Answer from the drawing. Dimensions are ordinates in mm from the lowest x, y and z of the part. A direction names the side the tool comes from. Give positions to 0.01 mm unless a question says otherwise; leave off trailing zeros. Write each loop counter-clockwise with the first axis right and the second up, starting at its lowest first coordinate (ties: lowest second). Pieces come first, ordered by that corner, then holes. Notation, with made-up numbers: (44.5, 55.25) -> (84.5, 55.25) arc R27 ccw to (84.5, 83.25) -> close; hole circle Ø2 at (3, 26). An arc over 180 degrees is marked (long way). Put each result on its own line as item: value. Start each with the question number.
1) Find the intervals of material crossed by line 1 along Y through (x, z) = (57, 10) (1 decimal); line 2 along Y through (x, z) = (55.95, 10.75) (1 decimal); line 3 along Z through (x, y) = (57, 18) (1 decimal), in increasing order. Write a range as from..to.
2) For the marked faces 1, 2 and 3, determine the directions among +Z, -Z, +X, -X, +Y, -Y from which every point of the face is accessible in a straight line to the end or side of a thin tool.
3) A cutting plane is placed at B-B (y = 27). Write down the section's boundary in (x, z), then the cut area to 3 significant figures.
4) A cutting plane is placed at A-A (z = 18.5). Write down the section's boundary in (x, y), then the cut area to 3 significant figures.
5) A cutting plane is placed at D-D (z = 3). Write down the section's boundary in (x, y), then the cut area to 3 significant figures.
6) A cutting plane is placed at C-C (x = 50). Write down the section's boundary in (y, z).
7) Flat-ended cylindrical pins translate along their axes: pin 1 Ø2.5 at (y, z) = (5.5, 11) entering from +X; pin 2 Ø0.6 at (x, y) = (3, 12.5) entering from -Z; pin 3 Ø4 at (y, z) = (5.08, 26.25) entering from -X. Find the tip coordinate at first contact, or state that the pin passes through.
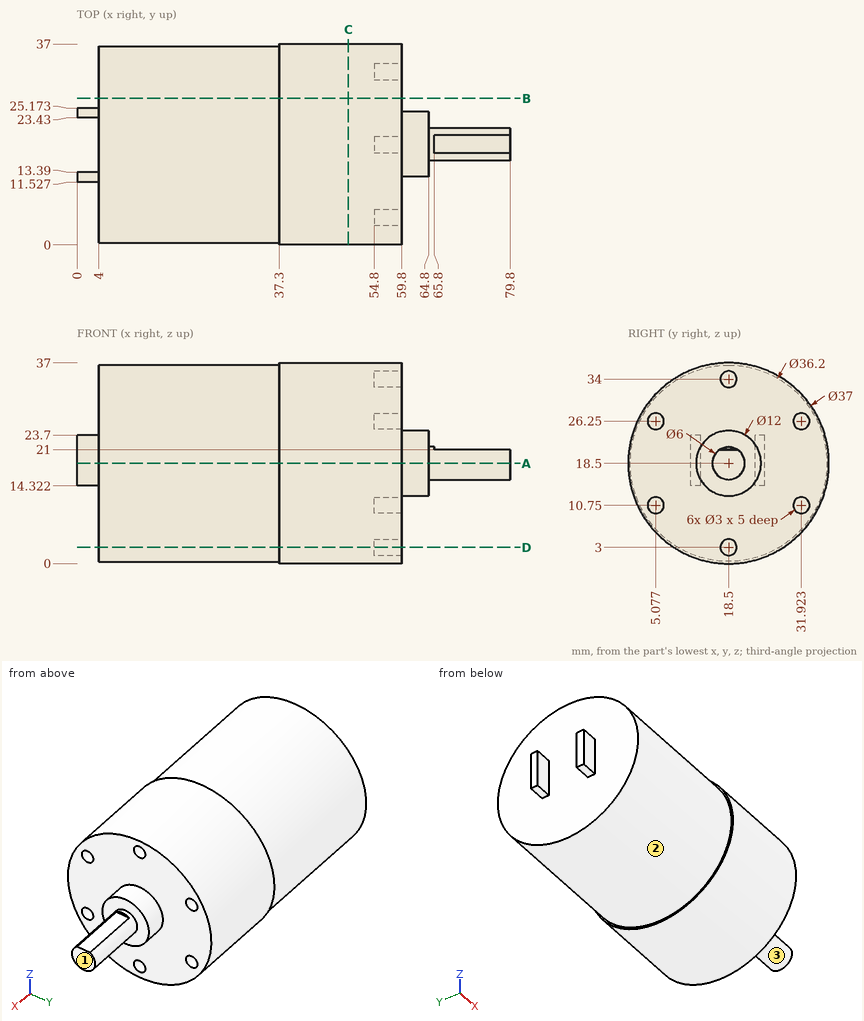
Reply:
1. line 1: y = 2.1..3.8, 6.4..30.6, 33.2..34.9
1. line 2: y = 1.7..3.6, 6.6..30.4, 33.4..35.3
1. line 3: z = 0..1.6, 4.4..32.6, 35.4..37
2. face 1: +Z, -Z, +X, +Y, -Y
2. face 2: -X
2. face 3: +X
3. outline: (4, 2.52) -> (37.3, 2.52) -> (37.3, 2.07) -> (59.8, 2.07) -> (59.8, 34.93) -> (37.3, 34.93) -> (37.3, 34.48) -> (4, 34.48) -> close
3. area: 1,800 mm2
4. outline: (0, 11.53) -> (4, 11.53) -> (4, 0.4) -> (37.3, 0.4) -> (37.3, 0) -> (59.8, 0) -> (59.8, 12.5) -> (64.8, 12.5) -> (64.8, 15.5) -> (79.8, 15.5) -> (79.8, 21.5) -> (64.8, 21.5) -> (64.8, 24.5) -> (59.8, 24.5) -> (59.8, 37) -> (37.3, 37) -> (37.3, 36.6) -> (4, 36.6) -> (4, 25.17) -> (0, 25.17) -> (0, 23.43) -> (4, 23.43) -> (4, 13.39) -> (0, 13.39) -> close
4. area: 2,200 mm2
5. outline: (4, 9.15) -> (37.3, 9.15) -> (37.3, 8.4) -> (59.8, 8.4) -> (59.8, 17) -> (54.8, 17) -> (54.8, 20) -> (59.8, 20) -> (59.8, 28.6) -> (37.3, 28.6) -> (37.3, 27.85) -> (4, 27.85) -> close
5. area: 1,060 mm2
6. outline: circle Ø37 at (18.5, 18.5)
7. pin 1: stops at x = 59.8
7. pin 2: stops at z = 14.32
7. pin 3: stops at x = 4
